Verification items for the finished model (mm, model axes). A direction names the side the tool comes from. Give positions to 0.01 mm unless a question says otherwise; leave off trailing zeros. Order: outer loops, then holes, each group sorted by start corner. A loop starts at its lowest first (then second) coordinate and runs counter-clockwise, first axis right, second up.
from build123d import *

# Parameters (mm, degrees)
F1_DEPTH = 203.2
F3_DEPTH = 25.4
F4_R     = 53.975
F5_DEPTH = 152.4
F4_R_2   = 9.525
F6_DEPTH = 76.2


with BuildPart() as f1:
    # F0 (on Front) → F1 (new body)
    with BuildSketch(Plane.XZ):
        Polygon((0, 177.8), (-203.2, 0), (203.2, 0), align=None)
    extrude(amount=F1_DEPTH)

    # F2 (on face) → F3 (cut)
    with BuildSketch(Plane.XZ.offset(203.2)):
        Polygon((0, 169.362322), (-193.556939, 0), (193.556939, 0), align=None)
    extrude(amount=-F3_DEPTH, mode=Mode.SUBTRACT)

    # F4 (on face) → F5 (cut)
    with BuildSketch(Plane.XZ.offset(177.8)):
        with Locations((0, 84.681161)):
            Circle(F4_R)
    extrude(amount=-F5_DEPTH, mode=Mode.SUBTRACT)

    # F4 (on face) → F6 (join)
    with BuildSketch(Plane.XZ.offset(177.8)):
        with Locations((0, 13.827616)):
            Circle(F4_R_2)
    extrude(amount=F6_DEPTH)


solid = f1.part
(1) Section check A-A, the plane z = 64. Enter the section's corners in (x, y), then the cut area to 3 significant figures.
Solved:
outline: (-130.06, -203.2) - (-120.41, -203.2) - (-120.41, -177.8) - (-49.86, -177.8) - (-49.86, -25.4) - (49.86, -25.4) - (49.86, -177.8) - (120.41, -177.8) - (120.41, -203.2) - (130.06, -203.2) - (130.06, 0) - (-130.06, 0) - close
area: 31,500 mm2
(2) Section check B-B, the plane x = 18.5. Enter the section's corners in (y, z), then the cut area to 3 significant figures.
Solved:
outline: (-203.2, 153.17) - (-177.8, 153.17) - (-177.8, 135.39) - (-25.4, 135.39) - (-25.4, 33.98) - (-177.8, 33.98) - (-177.8, 0) - (0, 0) - (0, 161.61) - (-203.2, 161.61) - close
area: 13,500 mm2
(3) Set-up check for faces 4 (the flat face through (-3, -100, 0)), 5 (the cylindrical face through (-2.06, -215.37, 4.53)): record each of +Z, -Z, +X, -X, +Y, -Y from which the full face is reachable in a straight line by a thin tool's end or side.
Solved:
face 4: -Z, +X, -X, +Y, -Y
face 5: -Y
(4) Scan lines: line 1 (Z direction, x = 0, y = -87); line 2 (Y direction, x = 6, z = 43.5); line 3 (Y direction, x = -13.5, z = 163). Record each from-to range of solid material in increasing order.
Solved:
line 1: z = 0 to 30.71, 138.66 to 177.8
line 2: y = -25.4 to 0
line 3: y = -203.2 to 0
(5) Release check for a two-part mould opening along Z. For faces 1 (the flat face through (-46, -203.2, 135)), 2 (the flat face through (-100.18, -100.18, 90.14)), 3 (the flat face through (-1, -25.4, 85)) record: pulls with the +Z half, pulls with the -Z half, needs draft (parallel to the pull), parting line crosses it, or undercut.
Solved:
face 1: needs draft
face 2: pulls with the +Z half
face 3: undercut
(6) Go/stop test with flat-tipped pins: pin 1 (4 mm diameter, centred on y = -43.5, z = 30.5, fed in from +X); pin 2 (4 mm diameter, centred on y = -149, z = 114.5, fed in from +X); pin 3 (1.5 mm diameter, centred on x = -1.5, z = 142.5, fed in from -Y); pin 4 (2 mm diameter, centred on x = 13.5, z = 128, fed in from +Y). Record where each tip stops, or that it passes through.
Solved:
pin 1: stops at x = 170.63
pin 2: stops at x = 74.63
pin 3: stops at y = -177.8
pin 4: stops at y = 0
(7) Section check C-C, the plane y = -131. Enter the section's corners in (x, z) (3 decimals).
Solved:
outline: (-203.2, 0) - (203.2, 0) - (0, 177.8) - close; hole circle Ø107.95 at (0, 84.681)
(8) Section check D-D, the plane z = 93. Enter the section's corners in (x, y), then the cut area to 3 significant figures.
Solved:
outline: (-96.91, -203.2) - (-87.27, -203.2) - (-87.27, -177.8) - (-53.33, -177.8) - (-53.33, -25.4) - (53.33, -25.4) - (53.33, -177.8) - (87.27, -177.8) - (87.27, -203.2) - (96.91, -203.2) - (96.91, 0) - (-96.91, 0) - close
area: 18,700 mm2
